Part model, mm, in its own coordinate system. A direction names the side the tool comes from. Coordinates: 2 decimals unless noted, no trailing zeros. Write each loop counter-clockwise with the first axis right and the second up, starting at its lowest first coordinate (ties: lowest second). Pieces come first, ordered by that corner, then holes. Notation, with made-up numbers: (83.5, 59) - (92.5, 59) arc R13 ccw to (92.5, 64) - close; hole circle Ø3 at (-22.75, 37). An arc over 180 degrees is marked (long way). Use a Markdown table: item, result.
```python
from build123d import *

# Parameters (mm, degrees)
PAD_DEPTH       = 2
SKETCH001_W     = 26
SKETCH001_H     = 2
PAD001_DEPTH    = 12
POCKET_DEPTH    = 5
SKETCH003_R     = 1.5
POCKET001_DEPTH = 5
CHAMFER_SIZE    = 2
CHAMFER001_SIZE = 1


with BuildPart() as part:
    # Sketch → Pad (new body)
    with BuildSketch(Plane.YZ):
        Polygon((0, 30), (0, 0), (26, 0), (26, 2), (21, 2), (5, 20), (5, 30), align=None)
    extrude(amount=PAD_DEPTH)

    # Sketch001 (on Face9 of Pad) → Pad001 (join)
    with BuildSketch(Plane.YZ.offset(2)):
        with Locations((13, 1)):
            Rectangle(SKETCH001_W, SKETCH001_H)
    extrude(amount=PAD001_DEPTH)

    # Sketch002 (on Face5 of Pad001) → Pocket (cut)
    with BuildSketch(Plane.YZ.offset(2)):
        with BuildLine():
            ThreePointArc((3.5, 26), (2.5, 27), (1.5, 26))
            Line((1.5, 26), (1.5, 6))
            ThreePointArc((1.5, 6), (2.5, 5), (3.5, 6))
            Line((3.5, 6), (3.5, 26))
        make_face()
    extrude(amount=-POCKET_DEPTH, mode=Mode.SUBTRACT)

    # Sketch003 (on Face16 of Pocket) → Pocket001 (cut)
    with BuildSketch(Plane(origin=(0, 0, 2), x_dir=(0, -1, 0), z_dir=(0, 0, 1))):
        with Locations((-22, 8)):
            Circle(SKETCH003_R)
        with Locations((-4, 8)):
            Circle(SKETCH003_R)
    extrude(amount=-POCKET001_DEPTH, mode=Mode.SUBTRACT)

    # Chamfer
    chamfer_edges = [part.edges().sort_by_distance(p)[0] for p in [
        (14, 0, 1),
        (14, 26, 1),
    ]]
    chamfer(chamfer_edges, length=CHAMFER_SIZE)

    # Chamfer001
    chamfer001_edges = [part.edges().sort_by_distance(p)[0] for p in [
        (1, 0, 30),
        (1, 5, 30),
    ]]
    chamfer(chamfer001_edges, length=CHAMFER001_SIZE)


solid = part.part
```
Item 1: Drill centre lines: probe 1 along X at (y, z) = (22, 0.55); probe 2 along Z at (x, y) = (3, 7.5). Where is each one in solid material? Low to high.
From the geometry:
| item | result |
|---|---|
| probe 1 | 0 to 6.5, 9.5 to 14 |
| probe 2 | 0 to 2 |
Item 2: Band-saw the part on C-C, the plane x = 10.75. Give the cut face in (y, z).
From the geometry:
| item | result |
|---|---|
| outline | (0, 0) - (26, 0) - (26, 2) - (0, 2) - close |
Item 3: Which spindle directions (+Z, -Z, +X, -X, +Y, -Y) get a long thin tool onto all of the face, cutting with end or side? Do faces 1 (the face through (1, 3, 30)), 2 (the face through (1, 2.5, 27)), 3 (the face through (2, 6, 10)). Say none if no direction does.
From the geometry:
| item | result |
|---|---|
| face 1 | +Z, +X, -X, +Y, -Y |
| face 2 | +X, -X |
| face 3 | +Z, +X, +Y, -Y |
Item 4: Drop flat-ended pins along their axis: P1, Ø6, axis at y = 9, z = 7, coming from the -X side; P2, Ø2, axis at x = 2.5, z = 12, coming from the +Y side; P3, Ø3.5, axis at x = 8, y = 4, coming from the +Z side; P4, Ø1.6, axis at x = 1, z = 15.5, coming from the +Y side. Give the stop position or say it passes through.
From the geometry:
| item | result |
|---|---|
| P1 | x = 0 |
| P2 | y = 12.88 |
| P3 | z = 2 |
| P4 | y = 9.71 |
Item 5: Band-saw the part on D-D, the plane y = 14. Give the cut face in (x, z) (3 decimals), then the cut area to 4 significant figures.
From the geometry:
| item | result |
|---|---|
| outline | (0, 0) - (14, 0) - (14, 2) - (2, 2) - (2, 9.875) - (0, 9.875) - close |
| area | 43.75 mm^2 |
Item 6: Band-saw the part on B-B, the plane x = 8. Give the cut face in (y, z).
From the geometry:
| item | result |
|---|---|
| outline | (0, 0) - (2.5, 0) - (2.5, 2) - (0, 2) - close; (5.5, 0) - (20.5, 0) - (20.5, 2) - (5.5, 2) - close; (23.5, 0) - (26, 0) - (26, 2) - (23.5, 2) - close |
Item 7: Band-saw the part on A-A, the plane y = 22. Give the cut face in (x, z).
From the geometry:
| item | result |
|---|---|
| outline | (0, 0) - (6.5, 0) - (6.5, 2) - (0, 2) - close; (9.5, 0) - (14, 0) - (14, 2) - (9.5, 2) - close |
Item 8: Two-plate mould, pull along Z, no slides. Class faces 4 (the face through (1, 0.5, 29.5)), 5 (the face through (1, 1.5, 16)), 6 (the face through (1, 2.5, 5)), 7 (the face through (1, 5, 24)): pulls with the +Z half, pulls with the -Z half, needs draft (parallel to the pull), parting line crosses it, or undercut.
From the geometry:
| item | result |
|---|---|
| face 4 | pulls with the +Z half |
| face 5 | undercut |
| face 6 | undercut |
| face 7 | needs draft |
